The model under review builds one solid part; all positions refer to its coordinate system, in mm. Face numbers are marked on the shaded views. A direction names the side the tool comes from. Round coordinates to 2 decimals unless told otherwise and drop trailing zeros. Order: outer loops, then holes, each group sorted by start corner. A loop starts at its lowest first (then second) coordinate and runs counter-clockwise, first axis right, second up. Notation, with made-up numbers: (1, 76.25) - (42, 76.25) arc R20 ccw to (42, 98.25) - close; hole circle Ø2 at (-25.5, 85). An arc over 180 degrees is marked (long way). One line per question, with ' | ' between items. Start each with the question number.
Item 1: Insertion check: pin 1 Ø5.5 at (x, z) = (4.2, 6.05) entering from +Y; pin 2 Ø8 at (y, z) = (-3.93, 6.02) entering from -X; pin 3 Ø3 at (y, z) = (-5.5, 6) entering from +X. Each pin has a flat end and moves straight along its axis. Give the tip position at first contact, or say it passes through.
Item 2: Draft analysis for pull direction X (two halves, no side actions). For the marked faces 3, 4, 5 and 6, state which applies: +X half, -X half, draft (parallel to the pull), parting line (faces both ways), or undercut.
Item 3: Add section D-D on z = 7. State the section outline as (x, y) points (3 decimals), and give its area (3 significant figures).
Item 4: Add section C-C on y = 3. State the section outline as (x, z) points.
Item 5: Add section B-B on x = -18. State the section outline as (y, z) points, and give its area (3 significant figures).
Item 6: Add section A-A on z = 12.75. State the section outline as (x, y) points.
Item 7: For L1, parallel to Y at x = -14, z = 14.5; L2, parallel to X at y = -14.5, z = 8.25; L3, parallel to Z at x = -12.5, y = 1, list the stretches that pass through material, from the lowest coordinate up. Write a range as [from, to].
Item 8: Tool access review of the marked faces 1 and 2: name each direction out of +Z, -Z, +X, -X, +Y, -Y from which nothing blocks a thin tool from reaching the whole face with its end or side.
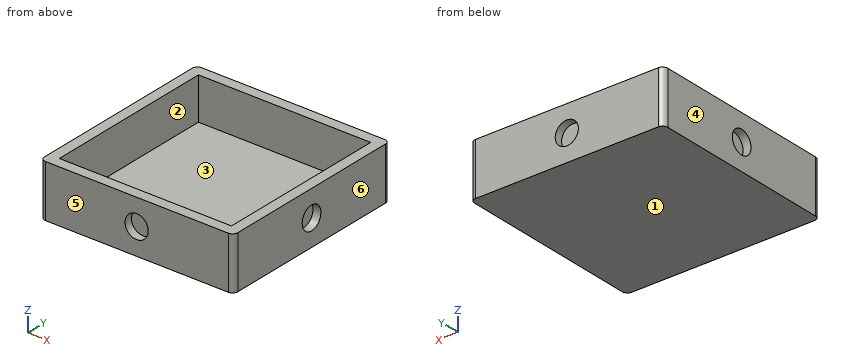
from build123d import *

# Parameters (mm, degrees)
F0_W        = 65.5
F0_H        = 65.5
F1_DEPTH    = 16
F2_T        = 4
F3_T1_DEPTH = 30
F4_R        = 4.4
F8_DEPTH    = 3
F9_DEPTH    = 3
F5_R        = 4.4
F10_DEPTH   = 3
F6_R        = 4.4
F11_DEPTH   = 3
F7_R        = 4.4
F12_DEPTH   = 3


# Not quite as in the source:
# - a fillet or chamfer that OpenCascade refuses, or shapes differently, is made with other operations: its cross-section is extruded or revolved along the edge and cut away or added


with BuildPart() as f1:
    # F0 (on Top) → F1 (new body)
    with BuildSketch(Plane.XY):
        with Locations((4.3041806072, -3.8802318871)):
            Rectangle(F0_W, F0_H)
    extrude(amount=F1_DEPTH)

    # F2
    f2_openings = [f1.faces().sort_by_distance(p)[0] for p in [
        (4.304181, -3.880232, 16),
    ]]
    offset(amount=F2_T, openings=f2_openings, kind=Kind.INTERSECTION)

    # F3: fillet of radius 2 on 4 edges, made by hand

    # F3_s2 → F3_t1 (cut)
    with BuildSketch(Plane.XY.offset(-9)):
        with BuildLine():
            ThreePointArc((41.0541806072, -38.6302318871), (40.4683941696, -40.0444454495), (39.0541806072, -40.6302318871))
            Line((39.0541806072, -40.6302318871), (41.0541806072, -40.6302318871))
            Line((41.0541806072, -40.6302318871), (41.0541806072, -38.6302318871))
        make_face()
        with BuildLine():
            ThreePointArc((41.0541806072, 30.8697681129), (40.4683941696, 32.2839816753), (39.0541806072, 32.8697681129))
            Line((39.0541806072, 32.8697681129), (41.0541806072, 32.8697681129))
            Line((41.0541806072, 32.8697681129), (41.0541806072, 30.8697681129))
        make_face()
        with BuildLine():
            ThreePointArc((-30.4458193928, 32.8697681129), (-31.8600329552, 32.2839816753), (-32.4458193928, 30.8697681129))
            Line((-32.4458193928, 30.8697681129), (-32.4458193928, 32.8697681129))
            Line((-32.4458193928, 32.8697681129), (-30.4458193928, 32.8697681129))
        make_face()
        with BuildLine():
            ThreePointArc((-32.4458193928, -38.6302318871), (-31.8600329552, -40.0444454495), (-30.4458193928, -40.6302318871))
            Line((-30.4458193928, -40.6302318871), (-32.4458193928, -40.6302318871))
            Line((-32.4458193928, -40.6302318871), (-32.4458193928, -38.6302318871))
        make_face()
    extrude(amount=F3_T1_DEPTH, mode=Mode.SUBTRACT)

    # F4 (on face) → F8 (join)
    with BuildSketch(Plane(origin=(-32.4458193928, 0, 0), x_dir=(0, -1, 0), z_dir=(-1, 0, 0))):
        with Locations((3.8802318871, 6)):
            Circle(F4_R)
    extrude(amount=-F8_DEPTH)

    # F4 (on face) → F9 (cut)
    with BuildSketch(Plane(origin=(-32.4458193928, 0, 0), x_dir=(0, -1, 0), z_dir=(-1, 0, 0))):
        with Locations((3.8802318871, 6)):
            Circle(F4_R)
    extrude(amount=-F9_DEPTH, mode=Mode.SUBTRACT)

    # F5 (on face) → F10 (cut)
    with BuildSketch(Plane.XZ.offset(40.6302318871)):
        with Locations((4.2000180173, 6.0547004089)):
            Circle(F5_R)
    extrude(amount=-F10_DEPTH, mode=Mode.SUBTRACT)

    # F6 (on face) → F11 (cut)
    with BuildSketch(Plane.YZ.offset(41.0541806072)):
        with Locations((-3.9293510383, 6.0207889489)):
            Circle(F6_R)
    extrude(amount=-F11_DEPTH, mode=Mode.SUBTRACT)

    # F7 (on face) → F12 (cut)
    with BuildSketch(Plane(origin=(0, 32.8697681129, 0), x_dir=(-1, 0, 0), z_dir=(0, 1, 0))):
        with Locations((-4.345219037, 6.0662772571)):
            Circle(F7_R)
    extrude(amount=-F12_DEPTH, mode=Mode.SUBTRACT)


solid = f1.part
Determined:
1) pin 1: y = 29.87 | pin 2: x = -29.45 | pin 3: x = 38.05
2) face 3: undercut | face 4: -X half | face 5: draft | face 6: +X half
3) outline: (-32.446, -38.63) arc R2 ccw to (-30.446, -40.63) - (-0.097, -40.63) - (-0.097, -37.63) - (8.497, -37.63) - (8.497, -40.63) - (39.054, -40.63) arc R2 ccw to (41.054, -38.63) - (41.054, -8.219) - (38.054, -8.219) - (38.054, 0.36) - (41.054, 0.36) - (41.054, 30.87) arc R2 ccw to (39.054, 32.87) - (8.645, 32.87) - (8.645, 29.87) - (0.045, 29.87) - (0.045, 32.87) - (-30.446, 32.87) arc R2 ccw to (-32.446, 30.87) - (-32.446, 0.405) - (-29.446, 0.405) - (-29.446, -8.165) - (-32.446, -8.165) - close; hole (-28.446, -36.63) - (37.054, -36.63) - (37.054, 28.87) - (-28.446, 28.87) - close | area: 1,010 mm2
4) outline: (-32.45, -4) - (41.05, -4) - (41.05, 16) - (37.05, 16) - (37.05, 0) - (-28.45, 0) - (-28.45, 16) - (-32.45, 16) - close
5) outline: (-40.63, -4) - (32.87, -4) - (32.87, 16) - (28.87, 16) - (28.87, 0) - (-36.63, 0) - (-36.63, 16) - (-40.63, 16) - close | area: 422 mm2
6) outline: (-32.45, -38.63) arc R2 ccw to (-30.45, -40.63) - (39.05, -40.63) arc R2 ccw to (41.05, -38.63) - (41.05, 30.87) arc R2 ccw to (39.05, 32.87) - (-30.45, 32.87) arc R2 ccw to (-32.45, 30.87) - close; hole (-28.45, -36.63) - (37.05, -36.63) - (37.05, 28.87) - (-28.45, 28.87) - close
7) L1: [-40.63, -36.63], [28.87, 32.87] | L2: [-32.45, -28.45], [37.05, 41.05] | L3: [-4, 0]
8) face 1: -Z, +X, -X, +Y, -Y | face 2: +Z
